Build history of the part. All positions in model axes, mm. A direction names the side the tool comes from. Give positions to 0.01 mm unless a question says otherwise; leave off trailing zeros. Loops run counter-clockwise (first coordinate to the right, second up) from the corner with the lowest first, then second, coordinate; pieces in that order, holes last.
1) Band-saw the part on B-B on z = 27. List the corners of the cut face in (x, y).
2) Band-saw the part on D-D on x = -31.75. List the corners of the cut face in (y, z), then the cut area to 3 significant figures.
3) Band-saw the part on C-C on y = 14. List the corners of the cut face in (x, z).
4) 3-axis set-ups, long thin cutter, end or side, ignore diameter. For faces 1 (the flat face through (-26, 26, 33.528)), 2 (the flat face through (-17, 31, 38.1)), 3 (the flat face through (-32, 7.874, 32)), 4 (the flat face through (-70, 32, 69.108)): which of +Z, -Z, +X, -X, +Y, -Y reach the whole face in a straight line?
5) Two-plate mould, pull along Y, no slides. Class faces 5 (the flat face through (-32, 55.626, 32)), 6 (the cylindrical face through (-69.761, 4.828, 61.407)), 7 (the flat face through (-6, 12.7, 3)), 8 (the flat face through (-16.002, 60, 32)): +Y half, -Y half, draft (parallel to the pull), parting line (faces both ways), or undercut.
6) Flat gauge pins, fed straight in: P1, Ø4, axis at x = -53, y = 19, coming from the +Z side; P2, Ø6.5, axis at x = -5, y = 41, coming from the -Z side; P3, Ø3, axis at y = 54.5, z = 44, coming from the +X side. Where does each tip first touch, or does it go through?
7) Band-saw the part on A-A on y = 31.75. List the corners of the cut face in (x, z), then the cut area to 3 significant figures.
8) Wall check: line 1 (Y direction, x = -31.75, z = 29); line 2 (Y direction, x = -31, z = 36); line 3 (X direction, y = 31, z = 34). Give the ranges that are in metal, low to high.
```python
from build123d import *

# Parameters (mm, degrees)
F0_W      = 31.75
F0_H      = 12.7
F0_W_2    = 15.748
F1_DEPTH  = 63.5
F2_DEPTH  = 7.874
F3_START  = -55.626
F3_DEPTH  = 7.874
F4_W      = 38.1
F4_H      = 6.35
F5_DEPTH  = 25.4
F6_R      = 12.7
F6_R_2    = 7.112
F7_DEPTH  = 4.572
F8_DEPTH  = 25.4
F10_DEPTH = 25.4
F11_DEPTH = 25.4


with BuildPart() as f1:
    # F0 (on Front) → F1 (new body)
    with BuildSketch(Plane.XZ):
        Polygon((-12.7, 0), (0, 0), (0, 38.1), (-16.002, 38.1), (-16.002, 25.4), (-12.7, 25.4), align=None)
        with Locations((-31.877, 31.75)):
            Rectangle(F0_W, F0_H)
        with Locations((-55.626, 31.75)):
            Rectangle(F0_W_2, F0_H)
        Polygon((-63.5, 25.4), (-63.5, 38.1), (-63.5, 73.9337697108), (-76.2, 73.9337697108), (-76.2, 25.4), align=None)
    extrude(amount=-F1_DEPTH)

    # F0 (on Front) → F2 (cut)
    with BuildSketch(Plane.XZ):
        with Locations((-31.877, 31.75)):
            Rectangle(F0_W, F0_H)
    extrude(amount=-F2_DEPTH, mode=Mode.SUBTRACT)

    # F0 (on Front) → F3 (cut)
    with BuildSketch(Plane.XZ.offset(F3_START)):
        with Locations((-31.877, 31.75)):
            Rectangle(F0_W, F0_H)
    extrude(amount=-F3_DEPTH, mode=Mode.SUBTRACT)

    # F4 (on face) → F5 (cut)
    with BuildSketch(Plane.YZ):
        with Locations((31.75, 3.175)):
            Rectangle(F4_W, F4_H)
    extrude(amount=-F5_DEPTH, mode=Mode.SUBTRACT)

    # F6 (on face) → F7 (cut)
    with BuildSketch(Plane.XY.offset(38.1)):
        with Locations((-31.75, 31.75)):
            Circle(F6_R)
        with Locations((-31.75, 31.75)):
            Circle(F6_R_2, mode=Mode.SUBTRACT)
    extrude(amount=-F7_DEPTH, mode=Mode.SUBTRACT)

    # F8 (cut): a face of the model
    f8_faces = [f1.faces().sort_by_distance(p)[0] for p in [
        (-31.75, 31.75, 38.1),
    ]]
    extrude(f8_faces, amount=-F8_DEPTH, mode=Mode.SUBTRACT)

    # F9 (on face) → F10 (cut)
    with BuildSketch(Plane.YZ.offset(-63.5)):
        with BuildLine():
            Line((63.5, 73.9337697108), (50.8, 73.9337697108))
            ThreePointArc((50.8, 73.9337697108), (59.7802561211, 70.2140258318), (63.5, 61.2337697108))
            Line((63.5, 61.2337697108), (63.5, 73.9337697108))
        make_face()
        with BuildLine():
            ThreePointArc((0, 61.2337697108), (3.7197438789, 70.2140258318), (12.7, 73.9337697108))
            Line((12.7, 73.9337697108), (0, 73.9337697108))
            Line((0, 73.9337697108), (0, 61.2337697108))
        make_face()
    extrude(amount=-F10_DEPTH, mode=Mode.SUBTRACT)

    # F9 (on face) → F11 (cut)
    with BuildSketch(Plane.YZ.offset(-63.5)):
        with BuildLine():
            Line((50.8, 69.1077697108), (12.7, 69.1077697108))
            ThreePointArc((12.7, 69.1077697108), (4.826, 61.2337697108), (12.7, 53.3597697108))
            Line((12.7, 53.3597697108), (50.8, 53.3597697108))
            ThreePointArc((50.8, 53.3597697108), (58.674, 61.2337697108), (50.8, 69.1077697108))
        make_face()
    extrude(amount=-F11_DEPTH, mode=Mode.SUBTRACT)


solid = f1.part
```
Findings below:
1. outline: (-76.2, 0) - (-47.75, 0) - (-47.75, 7.87) - (-16, 7.87) - (-16, 0) - (0, 0) - (0, 63.5) - (-16, 63.5) - (-16, 55.63) - (-47.75, 55.63) - (-47.75, 63.5) - (-76.2, 63.5) - close; hole circle Ø14.22 at (-31.75, 31.75)
2. outline: (7.87, 25.4) - (24.64, 25.4) - (24.64, 33.53) - (19.05, 33.53) - (19.05, 38.1) - (7.87, 38.1) - close; (38.86, 25.4) - (55.63, 25.4) - (55.63, 38.1) - (44.45, 38.1) - (44.45, 33.53) - (38.86, 33.53) - close
2. area: 375 mm2
3. outline: (-76.2, 25.4) - (-12.7, 25.4) - (-12.7, 6.35) - (0, 6.35) - (0, 38.1) - (-63.5, 38.1) - (-63.5, 53.36) - (-76.2, 53.36) - close; (-76.2, 69.11) - (-63.5, 69.11) - (-63.5, 73.93) - (-76.2, 73.93) - close
4. face 1: +Z
4. face 2: +Z, +X, +Y, -Y
4. face 3: +Z, -Z, -Y
4. face 4: +X, -X
5. face 5: +Y half
5. face 6: undercut
5. face 7: undercut
5. face 8: draft
6. P1: stops at z = 38.1
6. P2: stops at z = 6.35
6. P3: stops at x = -63.5
7. outline: (-76.2, 25.4) - (-38.86, 25.4) - (-38.86, 33.53) - (-44.45, 33.53) - (-44.45, 38.1) - (-63.5, 38.1) - (-63.5, 53.36) - (-76.2, 53.36) - close; (-76.2, 69.11) - (-63.5, 69.11) - (-63.5, 73.93) - (-76.2, 73.93) - close; (-24.64, 25.4) - (-12.7, 25.4) - (-12.7, 6.35) - (0, 6.35) - (0, 38.1) - (-19.05, 38.1) - (-19.05, 33.53) - (-24.64, 33.53) - close
7. area: 1,230 mm2
8. line 1: y = 7.87 to 24.64, 38.86 to 55.63
8. line 2: y = 7.87 to 19.07, 44.43 to 55.63
8. line 3: x = -76.2 to -44.43, -19.07 to 0
